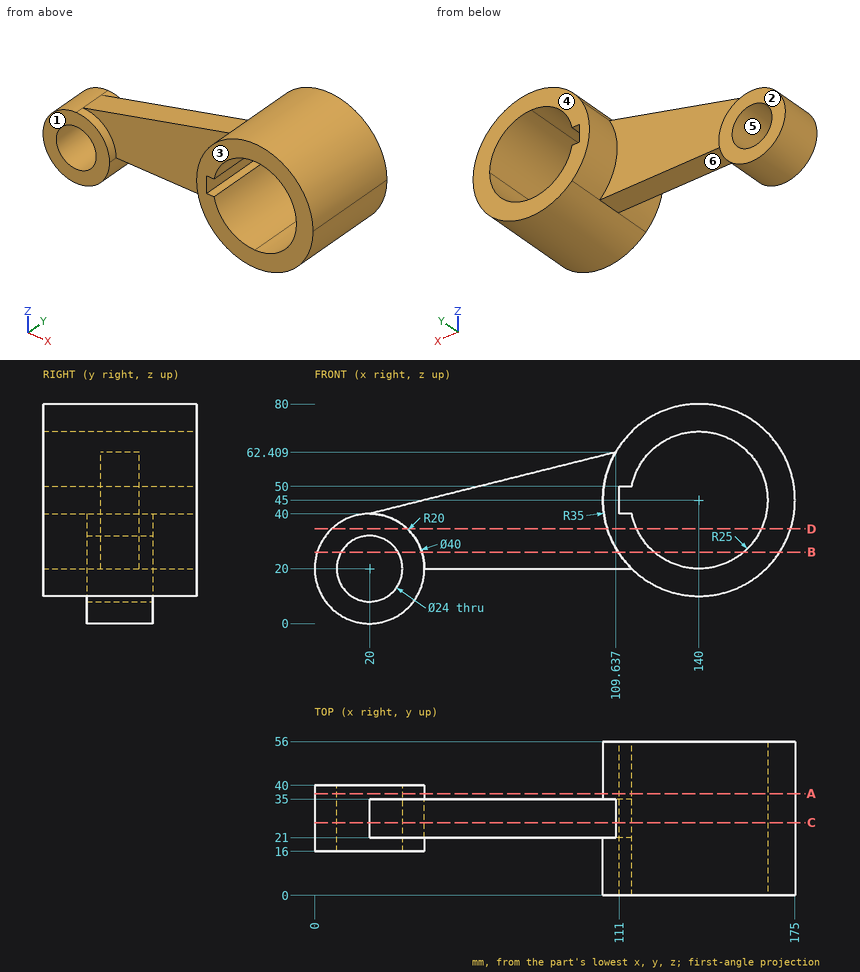
Design review of the part shown in the three views and the two pictorial views. Dimensions are in mm from the part's minimum x, y and z. A direction names the side the tool comes from. Coordinates: 2 decimals unless noted, no trailing zeros. Loops run counter-clockwise (first coordinate to the right, second up) from the corner with the lowest first, then second, coordinate; pieces in that order, holes last.
(1) Consider section B-B, the plane z = 26. Give the boundary of the cut face in (x, y).
Determined:
outline: (0.92, 16) - (9.61, 16) - (9.61, 40) - (0.92, 40) - close; (30.39, 16) - (39.08, 16) - (39.08, 21) - (110.61, 21) - (110.61, 0) - (123.75, 0) - (123.75, 56) - (110.61, 56) - (110.61, 35) - (39.08, 35) - (39.08, 40) - (30.39, 40) - close; (156.25, 0) - (169.39, 0) - (169.39, 56) - (156.25, 56) - close
(2) Consider section D-D, the plane z = 34.5. Give the boundary of the cut face in (x, y) (1 decimal), plus the area to 3 significant figures.
Determined:
outline: (6.2, 16) - (33.8, 16) - (33.8, 21) - (106.6, 21) - (106.6, 0) - (117.3, 0) - (117.3, 56) - (106.6, 56) - (106.6, 35) - (33.8, 35) - (33.8, 40) - (6.2, 40) - close; (162.7, 0) - (173.4, 0) - (173.4, 56) - (162.7, 56) - close
area: 2,880 mm2
(3) Insertion check: P1, Ø3, axis at y = 13.5, z = 61, coming from the -X side (1 decimal); P2, Ø1.4, axis at x = 113.5, y = 26.5, coming from the +Z side; P3, Ø1, axis at y = 35.5, z = 59, coming from the +X side; P4, Ø5, axis at y = 40, z = 46, coming from the +X side. Each pin has a flat end and moves straight along its axis. Give the tip position at first contact, or say it passes through.
Determined:
P1: stops at x = 108.1
P2: stops at z = 68.65
P3: stops at x = 172.29
P4: stops at x = 175
(4) Draft analysis for pull direction Z (two halves, no side actions). For the marked faces 4, 5 and 6, state which applies: +Z half, -Z half, draft (parallel to the pull), parting line (faces both ways), or undercut.
Determined:
face 4: draft
face 5: undercut
face 6: -Z half
(5) Consider section C-C, the plane y = 26.5. Give the boundary of the cut face in (x, z) (1 decimal).
Determined:
outline: (20, 40) arc R20 ccw (long way) to (40, 20) - (115.5, 20) arc R35 ccw (long way) to (109.6, 62.4) - close; hole circle Ø24 at (20, 20); hole (111, 40) - (115.5, 40) arc R25 ccw to (140, 20) arc R25 ccw to (140, 70) arc R25 ccw to (115.5, 50) - (111, 50) - close
(6) Consider section A-A, the plane y = 37. Give the boundary of the cut face in (x, z) (1 decimal), plus the area to 3 significant figures.
Determined:
outline: circle Ø40 at (20, 20); circle Ø70 at (140, 45); hole circle Ø24 at (20, 20); hole (111, 40) - (115.5, 40) arc R25 ccw to (140, 20) arc R25 ccw to (140, 70) arc R25 ccw to (115.5, 50) - (111, 50) - close
area: 2,650 mm2
(7) Tool access review of the marked faces 1, 2 and 3: name each direction out of +Z, -Z, +X, -X, +Y, -Y from which nothing blocks a thin tool from reaching the whole face with its end or side.
Determined:
face 1: +Z, -Z, -X, -Y
face 2: +Z, -Z, -X, +Y
face 3: +Z, -Z, +X, -X, -Y
(8) Wall thickness on L1, parallel to X at y = 26, z = 18; L2, parallel to X at y = 26.5, z = 17 (1 decimal); L3, parallel to Y at x = 73, z = 45: over which ranges is each line inside the solid? List them lowest first.
Determined:
L1: x = 0.1 to 8.17, 31.83 to 39.9, 117.73 to 162.27
L2: x = 0.2 to 8.4, 31.6 to 39.8, 119 to 161
L3: y = 21 to 35
